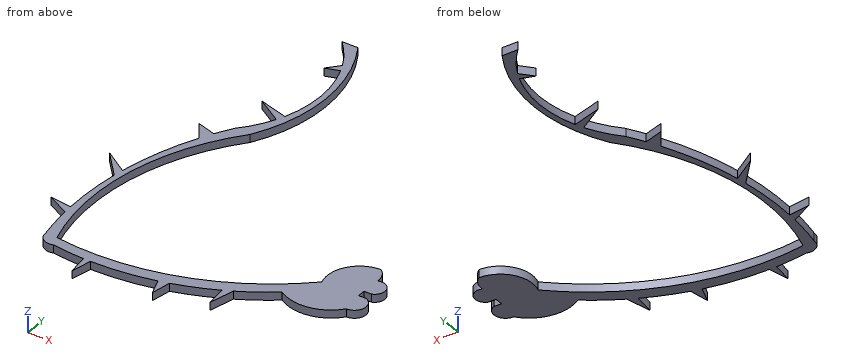
```python
from build123d import *

# Parameters (mm, degrees)
BOSS_EXTRUDE1_DEPTH = 1.524


with BuildPart() as part:
    # Sketch1 → Boss-Extrude1 (new body)
    with BuildSketch(Plane.XY):
        with BuildLine():
            Line((-6.707532294, -1.524), (-8.180261599, -1.524))
            Line((-8.180261599, -1.524), (-8.180261599, 0))
            Line((-8.180261599, 0), (-6.707532294, 0))
            ThreePointArc((-6.707532294, 0), (-5.566232372, 2.510291461), (-8.076523834, 3.651591383))
            ThreePointArc((-8.076523834, 3.651591383), (-8.369654544, 5.318155721), (-9.445515373, 6.624251346))
            ThreePointArc((-9.445515373, 6.624251346), (-14.401020029, 3.989835798), (-15.174514112, -1.568840176))
            ThreePointArc((-15.174514112, -1.568840176), (-34.4819371, -12.946344269), (-56.822290696, -14.716311235))
            ThreePointArc((-56.822290696, -14.716311235), (-57.967480091, 7.157863233), (-48.348408829, 26.836898663))
            ThreePointArc((-48.348408829, 26.836898663), (-44.246968405, 41.873579483), (-48.348408829, 56.910260303))
            Line((-48.348408829, 56.910260303), (-51.389474112, 56.910260303))
            ThreePointArc((-51.389474112, 56.910260303), (-49.216811045, 54.268914149), (-47.487026065, 51.318487362))
            Line((-47.487026065, 51.318487362), (-49.488434682, 49.065882941))
            Line((-49.488434682, 49.065882941), (-46.871051317, 49.924357948))
            ThreePointArc((-46.871051317, 49.924357948), (-45.319923788, 42.05338237), (-46.740158296, 34.157738817))
            Line((-46.740158296, 34.157738817), (-52.238150108, 35.775293633))
            Line((-52.238150108, 35.775293633), (-47.363457894, 32.688041845))
            ThreePointArc((-47.363457894, 32.688041845), (-49.134990292, 29.596317231), (-51.389474112, 26.836898663))
            ThreePointArc((-51.389474112, 26.836898663), (-52.30892636, 25.313565237), (-53.180617863, 23.762407254))
            Line((-53.180617863, 23.762407254), (-56.822290696, 24.868655134))
            Line((-56.822290696, 24.868655134), (-54.401149248, 21.377722623))
            ThreePointArc((-54.401149248, 21.377722623), (-57.245514929, 14.322290898), (-59.129790068, 6.952145706))
            Line((-59.129790068, 6.952145706), (-63.741523441, 10.016836401))
            Line((-63.741523441, 10.016836401), (-59.441762763, 5.107182625))
            ThreePointArc((-59.441762763, 5.107182625), (-60.018868287, -0.566291047), (-60.028931863, -6.26903188))
            Line((-60.028931863, -6.26903188), (-64.127892645, -5.71704549))
            Line((-64.127892645, -5.71704549), (-59.924854983, -7.930246527))
            ThreePointArc((-59.924854983, -7.930246527), (-59.56576898, -11.286860212), (-59.00955991, -14.616489269))
            ThreePointArc((-59.00955991, -14.616489269), (-58.101840622, -16.493067556), (-56.034305753, -16.759150133))
            ThreePointArc((-56.034305753, -16.759150133), (-53.001957218, -17.139391155), (-49.951949985, -17.332203884))
            Line((-49.951949985, -17.332203884), (-49.488434682, -21.174519893))
            Line((-49.488434682, -21.174519893), (-48.591597193, -17.35752957))
            ThreePointArc((-48.591597193, -17.35752957), (-42.573321797, -17.020849086), (-36.640297554, -15.956792779))
            Line((-36.640297554, -15.956792779), (-35.482848207, -19.212777207))
            Line((-35.482848207, -19.212777207), (-34.776442064, -15.465610409))
            ThreePointArc((-34.776442064, -15.465610409), (-30.729531902, -14.124143433), (-26.812740931, -12.440170747))
            Line((-26.812740931, -12.440170747), (-26.416692929, -16.322506345))
            Line((-26.416692929, -16.322506345), (-25.185933177, -11.619136315))
            ThreePointArc((-25.185933177, -11.619136315), (-21.861410327, -9.695823756), (-18.695636823, -7.521091244))
            ThreePointArc((-18.695636823, -7.521091244), (-12.816455315, -8.747608772), (-7.631399226, -5.71704549))
            ThreePointArc((-7.631399226, -5.71704549), (-5.42183259, -4.005584271), (-6.707532294, -1.524))
        make_face()
    extrude(amount=BOSS_EXTRUDE1_DEPTH)


solid = part.part
```
Input: part model. Units: mm. Frame: model coordinates. Give positions to 0.01 mm unless a question says otherwise; leave off trailing zeros. Order: outer loops, then holes, each group sorted by start corner. A loop starts at its lowest first (then second) coordinate and runs counter-clockwise, first axis right, second up.
1. Cut plane A-A (y = 40.5). Return loops of the section in (x, z), and give its area (3 significant figures).
Computed:
outline: (-45.36, 0) - (-44.28, 0) - (-44.28, 1.52) - (-45.36, 1.52) - close
area: 1.65 mm2
2. Cut plane B-B (x = -23.5). Return loops of the section in (y, z).
Computed:
outline: (-10.69, 0) - (-7.95, 0) - (-7.95, 1.52) - (-10.69, 1.52) - close
3. Pin query (flat end, axial travel): pin 1 Ø0.7 at (x, z) = (-7.5, 1) entering from -Y. Return the tip coordinate at first contact, or that it passes through.
Computed:
pin 1: stops at y = -5.98
4. Line query: probe 1 along Y at (x, z) = (-47, 0.3); probe 2 along Y at (x, z) = (-54, 1.3); probe 3 along X at (y, z) = (-11, 0.1). Output: solid intervals per line, ascending.
Computed:
probe 1: y = -17.34 to -15.2, 29.4 to 34.23, 49.88 to 54.34
probe 2: y = -17.04 to -15.05, 18.43 to 24.01
probe 3: x = -59.6 to -57.82, -29.33 to -24.05
